```python
from build123d import *

# Parameters (mm, degrees)
SKETCH_1_R      = 2.15
EXTRUDE_1_DEPTH = 3
CHAMFER_1_SIZE  = 2


with BuildPart() as part:
    # 草图1 → 凸台-拉伸1 (new body)
    with BuildSketch(Plane.XY):
        with BuildLine():
            Line((-61.5, 85.257359313), (-61.5, 39.742640687))
            ThreePointArc((-61.5, 39.742640687), (-61.728361402, 38.59459039), (-62.378679656, 37.621320344))
            Line((-62.378679656, 37.621320344), (-67.207106781, 32.792893219))
            ThreePointArc((-67.207106781, 32.792893219), (-67.423879533, 32.46846987), (-67.5, 32.085786438))
            Line((-67.5, 32.085786438), (-67.5, 5.414213562))
            ThreePointArc((-67.5, 5.414213562), (-67.423879533, 5.03153013), (-67.207106781, 4.707106781))
            Line((-67.207106781, 4.707106781), (-62.792893219, 0.292893219))
            ThreePointArc((-62.792893219, 0.292893219), (-62.46846987, 0.076120467), (-62.085786438, 0))
            Line((-62.085786438, 0), (62.085786438, 0))
            ThreePointArc((62.085786438, 0), (62.46846987, 0.076120467), (62.792893219, 0.292893219))
            Line((62.792893219, 0.292893219), (67.207106781, 4.707106781))
            ThreePointArc((67.207106781, 4.707106781), (67.423879533, 5.03153013), (67.5, 5.414213562))
            Line((67.5, 5.414213562), (67.5, 32.085786438))
            ThreePointArc((67.5, 32.085786438), (67.423879533, 32.46846987), (67.207106781, 32.792893219))
            Line((67.207106781, 32.792893219), (62.378679656, 37.621320344))
            ThreePointArc((62.378679656, 37.621320344), (61.728361402, 38.59459039), (61.5, 39.742640687))
            Line((61.5, 39.742640687), (61.5, 85.257359313))
            ThreePointArc((61.5, 85.257359313), (61.728361402, 86.40540961), (62.378679656, 87.378679656))
            Line((62.378679656, 87.378679656), (67.207106781, 92.207106781))
            ThreePointArc((67.207106781, 92.207106781), (67.423879533, 92.53153013), (67.5, 92.914213562))
            Line((67.5, 92.914213562), (67.5, 119.585786438))
            ThreePointArc((67.5, 119.585786438), (67.423879532, 119.96846987), (67.207106781, 120.292893219))
            Line((67.207106781, 120.292893219), (62.792893219, 124.707106781))
            ThreePointArc((62.792893219, 124.707106781), (62.46846987, 124.923879533), (62.085786438, 125))
            Line((62.085786438, 125), (-62.085786438, 125))
            ThreePointArc((-62.085786438, 125), (-62.46846987, 124.923879533), (-62.792893219, 124.707106781))
            Line((-62.792893219, 124.707106781), (-67.207106781, 120.292893219))
            ThreePointArc((-67.207106781, 120.292893219), (-67.423879533, 119.96846987), (-67.5, 119.585786438))
            Line((-67.5, 119.585786438), (-67.5, 92.914213562))
            ThreePointArc((-67.5, 92.914213562), (-67.423879533, 92.53153013), (-67.207106781, 92.207106781))
            Line((-67.207106781, 92.207106781), (-62.378679656, 87.378679656))
            ThreePointArc((-62.378679656, 87.378679656), (-61.728361402, 86.40540961), (-61.5, 85.257359313))
        make_face()
        with Locations((47.5, 10.25)):
            Circle(SKETCH_1_R, mode=Mode.SUBTRACT)
        with Locations((-47.5, 10.25)):
            Circle(SKETCH_1_R, mode=Mode.SUBTRACT)
        with Locations((-47.5, 114.75)):
            Circle(SKETCH_1_R, mode=Mode.SUBTRACT)
        with Locations((47.5, 114.75)):
            Circle(SKETCH_1_R, mode=Mode.SUBTRACT)
    extrude(amount=EXTRUDE_1_DEPTH)

    # 倒角1
    chamfer_1_edges = [part.edges().sort_by_distance(p)[0] for p in [
        (45.35, 10.25, 3),
        (-49.65, 10.25, 3),
        (-49.65, 114.75, 3),
        (45.35, 114.75, 3),
    ]]
    chamfer(chamfer_1_edges, length=CHAMFER_1_SIZE)


solid = part.part
```
Source: CAD feature listing. Evaluate the final solid. Frame: model axes, mm. A direction names the side the tool comes from. Round coordinates to 2 decimals unless told otherwise and drop trailing zeros. Write each loop counter-clockwise with the first axis right and the second up, starting at its lowest first coordinate (ties: lowest second). Pieces come first, ordered by that corner, then holes. Notation, with made-up numbers: M 44,-23 L 100,-23 A11 cw 100,-13 Z; hole C 54.5,49.25 d8. An arc over 180 degrees is marked long. Answer as a JSON object with one key per item and string values. Group by question number.
(1) Section query C-C on z = 2.55. State how many separate pieces and enclosed holes the cut face has, then the cut area to 3 significant figures.
(2) Section query D-D on y = 77. Output: boundary loops of the cut face in (x, z).
(3) Section query B-B on x = -47.5. Output: boundary loops of the cut face in (y, z).
(4) Reachability of faces 1 (the flat face through (65, 35, 1)), 2 (the flat face through (-61.5, 63, 1)), 3 (the cylindrical face through (49.55, 10.9, 0.49)) from +Z, -Z, +X, -X, +Y, -Y: full face, straight path, thin tool, end or side. Return the list, or none.
(5) First-contact query: pin 1 (7 mm diameter, centred on x = -47.5, y = 114.75, fed in from +Z); pin 2 (5 mm diameter, centred on x = 47.5, y = 114.75, fed in from -Z); pin 3 (4 mm diameter, centred on x = 47.5, y = 10.25, fed in from -Z). Flat tips, straight axial feed; report the tip coordinate or a pass-through.
(6) Ray query, line 1 (Y direction, x = 47.5, z = 0.65); line 2 (X direction, y = 8, z = 2.45); line 3 (Y direction, x = 47.5, z = 1.2). Return the intervals inside material, ascending. Write a range as [from, to].
(7) Mould query, pull axis Y, two halves, no side actions, for faces 4 (the conical face through (49.67, 115.433, 1.125)), 5 (the flat face through (65, 122.5, 1.5)), 6 (the flat face through (-67.5, 106, 1)). Classes: +Y half, -Y half, draft (parallel to the pull), parting line (faces both ways), or undercut.
(8) Section query A-A on y = 114.75. Output: boundary loops of the cut face in (x, z).
Computed values:
{
 "1": {"separate pieces": "1", "enclosed holes": "4", "area": "16,000 mm^2"},
 "2": {"outline": "M -61.5,0 L 61.5,0 L 61.5,3 L -61.5,3 Z"},
 "3": {"outline": "M 0,0 L 8.1,0 L 8.1,1 L 6.1,3 L 0,3 Z; M 12.4,0 L 112.6,0 L 112.6,1 L 110.6,3 L 14.4,3 L 12.4,1 Z; M 116.9,0 L 125,0 L 125,3 L 118.9,3 L 116.9,1 Z"},
 "4": {"face 1": "+Z, -Z, +X", "face 2": "+Z, -Z, -X", "face 3": "+Z, -Z"},
 "5": {"pin 1": "z = 2.35", "pin 2": "z = 0", "pin 3": "through"},
 "6": {"line 1": "[0, 8.1], [12.4, 112.6], [116.9, 125]", "line 2": "[-67.5, -50.31], [-44.69, 44.69], [50.31, 67.5]", "line 3": "[0, 7.9], [12.6, 112.4], [117.1, 125]"},
 "7": {"face 4": "undercut", "face 5": "+Y half", "face 6": "draft"},
 "8": {"outline": "M -67.5,0 L -49.65,0 L -49.65,1 L -51.65,3 L -67.5,3 Z; M -45.35,0 L 45.35,0 L 45.35,1 L 43.35,3 L -43.35,3 L -45.35,1 Z; M 49.65,0 L 67.5,0 L 67.5,3 L 51.65,3 L 49.65,1 Z"}
}
